from build123d import *

# Parameters (mm, degrees)
SKETCH1_R                = 14.9
BOSS_EXTRUDE1_DEPTH      = 27.7
SKETCH2_R                = 13.4
CUT_EXTRUDE1_DEPTH       = 10
BOSS_EXTRUDE2_DEPTH      = 3
BOSS_EXTRUDE2_DEPTH_BACK = 3
SKETCH3_W                = 15
SKETCH3_H                = 8
FILLET1_R                = 1


with BuildPart() as part:
    # Sketch1 → Boss-Extrude1 (new body)
    with BuildSketch(Plane(origin=(0, 0, 0), x_dir=(1, 0, 0), z_dir=(0, 1, 0))):
        with Locations(Location((0, 0, 0), (0, 0, 270))):
            Circle(SKETCH1_R)
    extrude(amount=BOSS_EXTRUDE1_DEPTH)

    # Sketch2 → Cut-Extrude1 (cut)
    with BuildSketch(Plane.XZ):
        with Locations(Location((0, 0, 0), (0, 0, 270))):
            Circle(SKETCH2_R)
    extrude(amount=-CUT_EXTRUDE1_DEPTH, mode=Mode.SUBTRACT)

    # Sketch3 → Boss-Extrude2 (add, two sides: drawn at the far end of the back side and taken through both)
    with BuildSketch(Plane.XY.offset(-BOSS_EXTRUDE2_DEPTH_BACK)):
        with Locations((0, 31.7)):
            Rectangle(SKETCH3_W, SKETCH3_H)
    extrude(amount=BOSS_EXTRUDE2_DEPTH + BOSS_EXTRUDE2_DEPTH_BACK)

    # Fillet1
    fillet1_edges = [part.edges().sort_by_distance(p)[0] for p in [
        (7.5, 27.7, 0),
        (0, 27.7, -3),
        (-7.5, 27.7, 0),
        (0, 27.7, 3),
    ]]
    fillet(fillet1_edges, radius=FILLET1_R)


solid = part.part
Geometry: final body of the model. Coordinates: model frame, mm. A direction names the side the tool comes from. Round coordinates to 2 decimals unless told otherwise and drop trailing zeros. Write each loop counter-clockwise with the first axis right and the second up, starting at its lowest first coordinate (ties: lowest second). Pieces come first, ordered by that corner, then holes. Notation, with made-up numbers: M 21.5,-26 L 26.5,-26 A9 cw 26.5,-18 Z; hole C -4,50.5 d5. An arc over 180 degrees is marked long. Write item = value, one per line.
Item 1: Section query B-B on x = 0. Return loops of the section in (y, z).
Findings:
outline = M 0,-14.9 L 27.7,-14.9 L 27.7,-4 A1 cw 28.7,-3 L 35.7,-3 L 35.7,3 L 28.7,3 A1 cw 27.7,4 L 27.7,14.9 L 0,14.9 L 0,13.4 L 10,13.4 L 10,-13.4 L 0,-13.4 Z
Item 2: Material intervals for line 1 along X through (y, z) = (6.25, 0); line 2 along Y through (x, z) = (0.25, 12.5); line 3 along X through (y, z) = (2, -8.5), sorted ascending. Write a range as [from, to].
Findings:
line_1 = [-14.9, -13.4], [13.4, 14.9]
line_2 = [10, 27.7]
line_3 = [-12.24, -10.36], [10.36, 12.24]
Item 3: Pull-direction query (X, two-part tool) for faces 6 (the face through (0, 10, 0)), 7 (the face through (-7.5, 32, 0)), 8 (the face through (0, 32, 3)); classes: pulls with the +X half, pulls with the -X half, needs draft (parallel to the pull), parting line crosses it, or undercut.
Findings:
face_6 = undercut
face_7 = pulls with the -X half
face_8 = needs draft
Item 4: Section query C-C on y = 6.5. Return loops of the section in (x, z), then the cut area to 3 significant figures.
Findings:
outline = C 0,0 d29.8; hole C 0,0 d26.8
area = 133 mm^2
Item 5: Section query A-A on z = 0. Return loops of the section in (x, y), then the cut area to 3 significant figures.
Findings:
outline = M -14.9,0 L -13.4,0 L -13.4,10 L 13.4,10 L 13.4,0 L 14.9,0 L 14.9,27.7 L 8.5,27.7 A1 cw 7.5,28.7 L 7.5,35.7 L -7.5,35.7 L -7.5,28.7 A1 cw -8.5,27.7 L -14.9,27.7 Z
area = 678 mm^2
Item 6: Access query for faces 1 (the face through (-8.2, 4.9, 10.6)), 2 (the face through (0, 27.7, 6)), 3 (the face through (0, 32, -3)), 4 (the face through (7.5, 32, 0)), 5 (the face through (0.119, 27.985, 3.301)). Directions: +Z, -Z, +X, -X, +Y, -Y. A direction counts if a zero-diameter tool reaches every point of the face in a straight line with its end or side. Return the directions, or none.
Findings:
face_1 = -Y
face_2 = +Y
face_3 = -Z, +X, -X, +Y
face_4 = +Z, -Z, +X, +Y
face_5 = +Z, +X, -X, +Y
Item 7: Section query D-D on y = 33. Return loops of the section in (x, z), then the cut area to 3 significant figures.
Findings:
outline = M -7.5,-3 L 7.5,-3 L 7.5,3 L -7.5,3 Z
area = 90.0 mm^2
Item 8: Pin query (flat end, axial travel): P1, Ø2, axis at y = 29.5, z = -2, coming from the -X side; P2, Ø7.5, axis at x = -2.5, y = 33, coming from the +Z side; P3, Ø6, axis at x = -10.5, y = 17.5, coming from the -Z side. Return the tip coordinate at first contact, or that it passes through.
Findings:
P1 = -7.52
P2 = 3
P3 = -12.87
